```python
from build123d import *

# Parameters (mm, degrees)
CYLINDER002_R     = 3
CYLINDER002_DEPTH = 3
CYLINDER001_R     = 1.7
CYLINDER001_DEPTH = 25


with BuildPart() as cylinder002:
    # Cylinder002 → Cylinder002 (new body)
    with BuildSketch(Plane.XY):
        Circle(CYLINDER002_R)
    extrude(amount=CYLINDER002_DEPTH)


with BuildPart() as screw:
    # Cylinder001 → Cylinder001 (new body)
    with BuildSketch(Plane.XY):
        Circle(CYLINDER001_R)
    extrude(amount=CYLINDER001_DEPTH)

    # Fusion: union Cylinder002
    add(cylinder002.part)


solid = screw.part
```
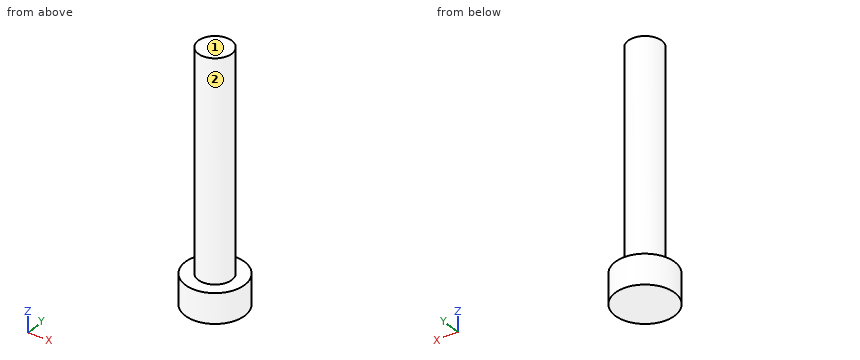
Geometry check sheet. Reference: the model listing, model coordinates, mm. Face numbers are marked on the shaded views. A direction names the side the tool comes from. Coordinates: 2 decimals unless noted, no trailing zeros. Write each loop counter-clockwise with the first axis right and the second up, starting at its lowest first coordinate (ties: lowest second). Pieces come first, ordered by that corner, then holes. Notation, with made-up numbers: M 56.25,4.5 L 61.25,4.5 A26 cw 61.25,22.5 Z; hole C 70,16.25 d7. An arc over 180 degrees is marked long. One line per item, written item: value. Start each with the question number.
(1) Sectioned sample at D-D, the plane y = -2.1. Enter the section's corners in (x, z), and give its area (3 significant figures).
(2) Depth check by flat-ended pin: pin 1 (1.5 mm diameter, centred on y = 0.5, z = 21, fed in from -X); pin 2 (2 mm diameter, centred on x = 2, z = 9.5, fed in from -Y). Enter the tip coordinate at first touch or a pass-through.
(3) Scan lines: line 1 along Z through (x, y) = (-0.4, 2.3); line 2 along Y through (x, z) = (-0.1, 1); line 3 along X through (y, z) = (-1, 8). Record each from-to range of solid material in increasing order. Write a range as [from, to].
(4) Sectioned sample at C-C, the plane z = 18.25. Enter the section's corners in (x, y), and give its area (3 significant figures).
(5) Tool access check on the marked faces 1 and 2. Record the directions out of +Z, -Z, +X, -X, +Y, -Y that give a thin tool (end or side, any length) a straight path to the whole face; none if there is none.
(6) Sectioned sample at A-A, the plane x = 0. Enter the section's corners in (y, z), and give its area (3 significant figures).
Filled sheet:
1. outline: M -2.14,0 L 2.14,0 L 2.14,3 L -2.14,3 Z
1. area: 12.9 mm²
2. pin 1: x = -1.7
2. pin 2: y = -1.37
3. line 1: [0, 3]
3. line 2: [-3, 3]
3. line 3: [-1.37, 1.37]
4. outline: C 0,0 d3.4
4. area: 9.08 mm²
5. face 1: +Z, +X, -X, +Y, -Y
5. face 2: +Z
6. outline: M -3,0 L 3,0 L 3,3 L 1.7,3 L 1.7,25 L -1.7,25 L -1.7,3 L -3,3 Z
6. area: 92.8 mm²
